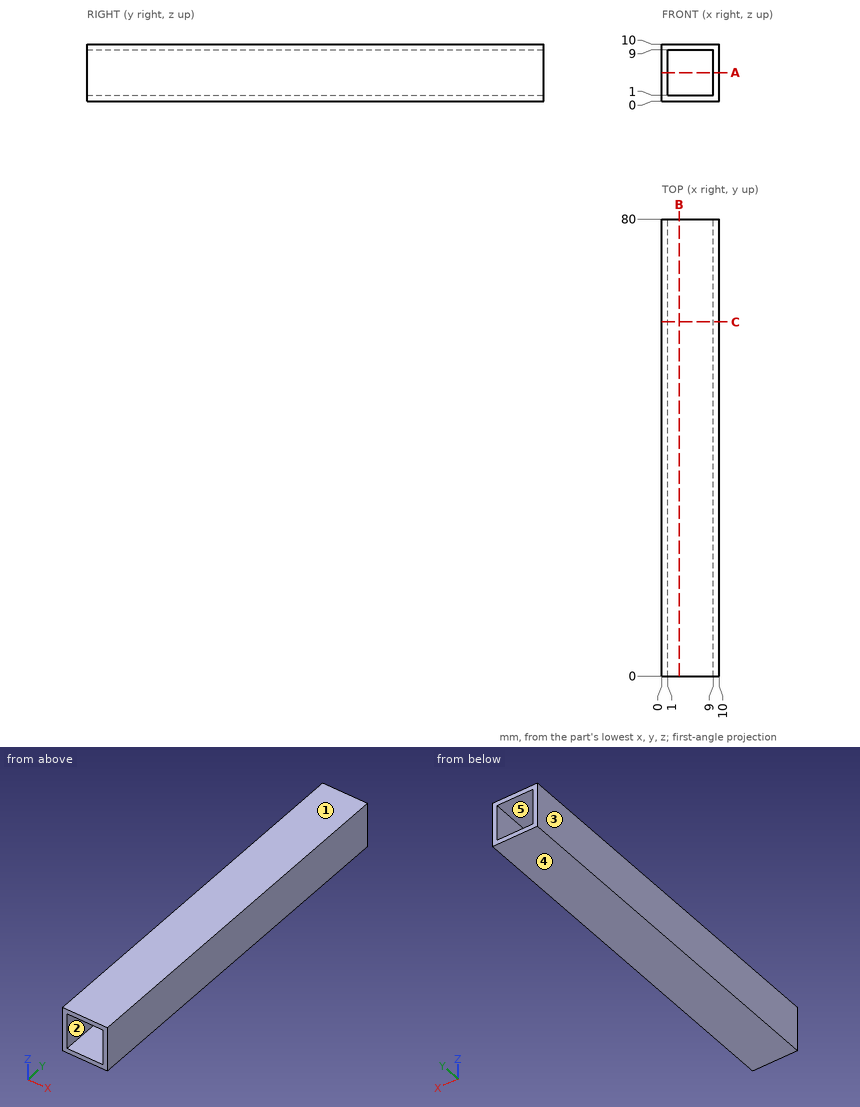
Design review of the part shown in the three views and the two pictorial views. Dimensions are in mm from the part's minimum x, y and z. A direction names the side the tool comes from. Round coordinates to 2 decimals unless told otherwise and drop trailing zeros. Write each loop counter-clockwise with the first axis right and the second up, starting at its lowest first coordinate (ties: lowest second). Pieces come first, ordered by that corner, then holes.
Item 1: Draft analysis for pull direction Z (two halves, no side actions). For the marked faces 1, 2 and 3, state which applies: released by +Z, released by -Z, zero draft, split by the parting line, or undercut.
Item 2: Consider section A-A on z = 5. Give the boundary of the cut face in (x, y).
Item 3: Consider section B-B on x = 3. Give the boundary of the cut face in (y, z), and give its area (3 significant figures).
Item 4: Wall thickness on L1, parallel to X at y = 70, z = 3.5: over which ranges is the line inside the solid? List them lowest first.
Item 5: Consider section C-C on y = 62. Give the boundary of the cut face in (x, z).
Item 6: For the marked faces 4 and 5, list the 3-axis set-ups (+Z, -Z, +X, -X, +Y, -Y) from which the entire face can be reached by the end or side of a thin tool; tool diameter is ignored.
Item 7: For pin 1 Ø1 at (x, z) = (4, 3) entering from -Y, flat-tipped, find the tip position at first contact; note if it passes through.
Check values:
1. face 1: released by +Z
1. face 2: undercut
1. face 3: zero draft
2. outline: (0, 0) - (1, 0) - (1, 80) - (0, 80) - close; (9, 0) - (10, 0) - (10, 80) - (9, 80) - close
3. outline: (0, 0) - (80, 0) - (80, 1) - (0, 1) - close; (0, 9) - (80, 9) - (80, 10) - (0, 10) - close
3. area: 160 mm2
4. L1: x = 0 to 1, 9 to 10
5. outline: (0, 0) - (10, 0) - (10, 10) - (0, 10) - close; hole (1, 1) - (9, 1) - (9, 9) - (1, 9) - close
6. face 4: -Z, +X, -X, +Y, -Y
6. face 5: +Y, -Y
7. pin 1: passes through
